Design review of the part built by this model. Coordinates are the model's own, in mm. Face numbers are marked on the shaded views. Coordinates: 2 decimals unless noted, no trailing zeros. Loops run counter-clockwise (first coordinate to the right, second up) from the corner with the lowest first, then second, coordinate; pieces in that order, holes last. Notation, with made-up numbers: (0, 52.25) -> (55, 52.25) arc R26 cw to (55, 81.25) -> close; hole circle Ø9 at (68, 78.25). An arc over 180 degrees is marked (long way). One line per item, written item: value. Start each with the question number.
1. Insertion check: pin 1 (1 mm diameter, centred on x = -7.5, y = -16, fed in from -Z). The pin has a flat end and moves straight along its axis. Give the tip position at first contact, or say it passes through.
2. Add section B-B on x = -8.5. Write out the cut boundary in (y, z), plus the area to 3 significant figures.
3. For probe 1 along Z at (x, y) = (-8.5, -17); probe 2 along X at (y, z) = (-11, 25); probe 3 along Z at (x, y) = (-9, -15.5), list the stretches that pass through material, from the lowest coordinate up.
4. Add section C-C on y = -7.25. Write out the cut boundary in (x, z) (3 decimals).
5. Add section A-A on z = 23. Write out the cut boundary in (x, y).
6. Draft analysis for pull direction X (two halves, no side actions). For the marked faces 1, 2 and 3, state which applies: pulls with the +X half, pulls with the -X half, needs draft (parallel to the pull), parting line crosses it, or undercut.
7. Add section D-D on z = 10. Write out the cut boundary in (x, y).
```python
from build123d import *

# Parameters (mm, degrees)
F0_W      = 17
F0_H      = 50
F1_DEPTH  = 18
F3_D      = 5
F3_DEPTH  = 25
F3_TIP    = 1.5021515476
F5_DEPTH  = 25
F6_R      = 9.5
F7_DEPTH  = 25
F8_R      = 9.5
F8_R_2    = 1.6285775441
F9_DEPTH  = 25
F10_R     = 9.5
F11_DEPTH = 25
F12_SIZE  = 2


with BuildPart() as f1:
    # F0 (on Front) → F1 (new body)
    with BuildSketch(Plane.XZ):
        with Locations((-8.5, 25)):
            Rectangle(F0_W, F0_H)
    extrude(amount=F1_DEPTH)

    # F3
    with Locations(Plane.XZ.offset(18)):
        with Locations((-8.5, 10), (-8.5, 25)):
            Hole(F3_D / 2, depth=F3_DEPTH)
            with Locations((0, 0, -(F3_DEPTH + F3_TIP / 2))):  # 118° drill point
                Cone(0, F3_D / 2, F3_TIP, mode=Mode.SUBTRACT)

    # F4 (on face) → F5 (cut)
    with BuildSketch(Plane(origin=(-17, 0, 0), x_dir=(0, -1, 0), z_dir=(-1, 0, 0))):
        Polygon((0, 50), (0, 8), (12, 50), align=None)
    extrude(amount=-F5_DEPTH, mode=Mode.SUBTRACT)

    # F6 (on Front) → F7 (cut)
    with BuildSketch(Plane.XZ):
        with Locations((-8.5753183812, -6.7173321731)):
            Circle(F6_R)
    extrude(amount=-F7_DEPTH, mode=Mode.SUBTRACT)

    # F8 (on Front) → F9 (cut)
    with BuildSketch(Plane.XZ):
        with Locations((-8.2726162836, -6.7173321731)):
            Circle(F8_R)
        with Locations((10.9988851703, -6.7173321731)):
            Circle(F8_R_2)
    extrude(amount=-F9_DEPTH, mode=Mode.SUBTRACT)

    # F10 (on face) → F11 (cut)
    with BuildSketch(Plane(origin=(0, 0, 0), x_dir=(-1, 0, 0), z_dir=(0, 1, 0))):
        with Locations((8.5753183812, -6.4314883202)):
            Circle(F10_R)
        with BuildLine():
            Line((1.5834689844, 0), (15.5671677779, 0))
            ThreePointArc((15.5671677779, 0), (8.5753183812, 3.0685116798), (1.5834689844, 0))
        make_face()
    extrude(amount=-F11_DEPTH, mode=Mode.SUBTRACT)

    # F12
    f12_edges = [f1.edges().sort_by_distance(p)[0] for p in [
        (0, -6, 29),
        (-17, -6, 29),
    ]]
    chamfer(f12_edges, length=F12_SIZE)


solid = f1.part
```
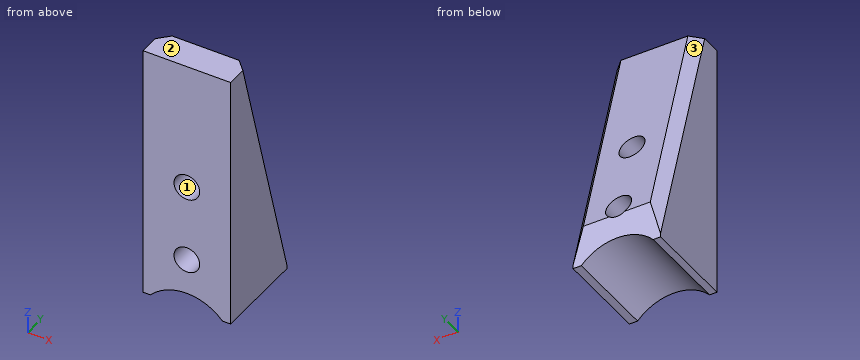
Worked answers:
1. pin 1: stops at z = 2.94
2. outline: (-18, 3.07) -> (0, 3.07) -> (0, 7.5) -> (-18, 7.5) -> close; (-18, 12.5) -> (-1.29, 12.5) -> (-4.14, 22.5) -> (-18, 22.5) -> close; (-18, 27.5) -> (-5.57, 27.5) -> (-12, 50) -> (-18, 50) -> close
2. area: 440 mm²
3. probe 1: z = 3.07 to 7.5, 12.5 to 22.5, 27.5 to 50
3. probe 2: x = -17 to -11, -6 to 0
3. probe 3: z = 3.06 to 7.55, 12.45 to 22.55, 27.45 to 50
4. outline: (-17, 0) -> (-15.567, 0) arc R9.5 cw to (-1.583, 0) -> (0, 0) -> (0, 26.095) -> (-2, 33.375) -> (-15, 33.375) -> (-17, 26.095) -> close; hole circle Ø5 at (-8.5, 10); hole circle Ø5 at (-8.5, 25)
5. outline: (-17, -18) -> (-10, -18) -> (-10, -4.29) -> (-15, -4.29) -> (-17, -6.37) -> close; (-7, -18) -> (0, -18) -> (0, -6.37) -> (-2, -4.29) -> (-7, -4.29) -> close
6. face 1: undercut
6. face 2: needs draft
6. face 3: pulls with the -X half
7. outline: (-17, -18) -> (-11, -18) -> (-11, -0.57) -> (-15, -0.57) -> (-17, -2.65) -> close; (-6, -18) -> (0, -18) -> (0, -2.65) -> (-2, -0.57) -> (-6, -0.57) -> close
